For this review, take the finished solid that the model builds, in its own axes (mm). Face numbers are marked on the shaded views. A direction names the side the tool comes from. Give positions to 0.01 mm unless a question says otherwise; leave off trailing zeros. Order: outer loops, then holes, each group sorted by start corner. A loop starts at its lowest first (then second) coordinate and runs counter-clockwise, first axis right, second up. Notation, with made-up numbers: (46.25, 45.5) - (56.25, 45.5) arc R24 cw to (56.25, 65.5) - close; hole circle Ø11 at (84, 30.5). An arc over 180 degrees is marked (long way). One line per item, written item: value.
```python
from build123d import *

# Parameters (mm, degrees)
SKETCH_1_R                   = 36
EXTRUDE_1_DEPTH              = 26.5
CUT_EXTRUDE_3_DEPTH          = 58.395557319
CUT_EXTRUDE_3_DEPTH_BACK     = 58.395557319
SKETCH_5_R                   = 24
CUT_EXTRUDE_4_DEPTH          = 74.491496107
CUT_EXTRUDE_4_DEPTH_BACK     = 74.491496107
CUT_EXTRUDE_2_DEPTH          = 21.5
HOLE_WIZARD_M3_1_D           = 3.4
HOLE_WIZARD_M3_1_DEPTH       = 5
HOLE_WIZARD_M3_1_CBORE_D     = 6.5
HOLE_WIZARD_M3_1_CBORE_DEPTH = 3
PATTERN_CIRCULAR_1_COUNT     = 2
PATTERN_CIRCULAR_1_ANGLE     = 45
F_1_THE_OTHER_WAY_COUNT      = 2
F_1_THE_OTHER_WAY_ANGLE      = 45
MIRROR_1_COPY_1_D            = 3.4
MIRROR_1_COPY_1_DEPTH        = 5
MIRROR_1_COPY_1_CBORE_D      = 6.5
MIRROR_1_COPY_1_CBORE_DEPTH  = 3
MIRROR_1_COPY_2_D            = 3.4
MIRROR_1_COPY_2_DEPTH        = 5
MIRROR_1_COPY_2_CBORE_D      = 6.5
MIRROR_1_COPY_2_CBORE_DEPTH  = 3
FILLET_1_R                   = 5
SKETCH_10_R                  = 17.5
EXTRUDE_2_DEPTH              = 5
SKETCH_17_R                  = 15
EXTRUDE_3_DEPTH              = 7


with BuildPart() as part:
    # ｽｹｯﾁ1 → ﾎﾞｽ - 押し出し1 (new, symmetric)
    with BuildSketch(Plane.XY):
        Circle(SKETCH_1_R)
    extrude(amount=EXTRUDE_1_DEPTH, both=True)

    # ｽｹｯﾁ5 → ｶｯﾄ - 押し出し3 (cut, two sides: drawn at the far end of the back side and taken through both)
    with BuildSketch(Plane.XY.offset(-CUT_EXTRUDE_3_DEPTH_BACK)):
        Circle(SKETCH_5_R)
    extrude(amount=CUT_EXTRUDE_3_DEPTH + CUT_EXTRUDE_3_DEPTH_BACK, mode=Mode.SUBTRACT)

    # ｽｹｯﾁ6 → ｶｯﾄ - 押し出し4 (cut, two sides: drawn at the far end of the back side and taken through both)
    with BuildSketch(Plane.XY.offset(26.5).offset(-CUT_EXTRUDE_4_DEPTH_BACK)):
        with BuildLine():
            Line((-33.25966317, 13.776603565), (0, 0))
            Line((0, 0), (33.25966317, 13.776603565))
            ThreePointArc((33.25966317, 13.776603565), (0, -36), (-33.25966317, 13.776603565))
        make_face()
    extrude(amount=CUT_EXTRUDE_4_DEPTH + CUT_EXTRUDE_4_DEPTH_BACK, mode=Mode.SUBTRACT)

    # ｽｹｯﾁ3 → ｶｯﾄ - 押し出し2 (cut, symmetric)
    with BuildSketch(Plane.XY):
        with BuildLine():
            Line((-33.25966317, 13.776603565), (-28.640265508, 11.863186403))
            ThreePointArc((-28.640265508, 11.863186403), (0, 31), (28.640265508, 11.863186403))
            Line((28.640265508, 11.863186403), (33.25966317, 13.776603565))
            ThreePointArc((33.25966317, 13.776603565), (0, -36), (-33.25966317, 13.776603565))
        make_face()
    extrude(amount=CUT_EXTRUDE_2_DEPTH, both=True, mode=Mode.SUBTRACT)

    # M3 穴付きねじ用座ぐり穴1
    with Locations(Plane.XY.offset(26.5)):
        with Locations((0, 27.5)):
            hole_wizard_m3_1 = CounterBoreHole(HOLE_WIZARD_M3_1_D / 2, HOLE_WIZARD_M3_1_CBORE_D / 2, HOLE_WIZARD_M3_1_CBORE_DEPTH, depth=HOLE_WIZARD_M3_1_DEPTH)

    # 円形ﾊﾟﾀｰﾝ1: M3 穴付きねじ用座ぐり穴1 ×2 about axis
    pattern_circular_1_axis = Axis((0, 0, 26.5), (0, 0, -1))
    for i in range(1, PATTERN_CIRCULAR_1_COUNT):
        add(hole_wizard_m3_1.rotate(pattern_circular_1_axis, i * PATTERN_CIRCULAR_1_ANGLE / (PATTERN_CIRCULAR_1_COUNT - 1)), mode=Mode.SUBTRACT)

    # 1 the other way: M3 穴付きねじ用座ぐり穴1 ×2 about axis
    f_1_the_other_way_axis = Axis((0, 0, 26.5), (0, 0, 1))
    for i in range(1, F_1_THE_OTHER_WAY_COUNT):
        add(hole_wizard_m3_1.rotate(f_1_the_other_way_axis, i * F_1_THE_OTHER_WAY_ANGLE / (F_1_THE_OTHER_WAY_COUNT - 1)), mode=Mode.SUBTRACT)

    # ﾐﾗｰ1: M3 穴付きねじ用座ぐり穴1 across plane
    add(hole_wizard_m3_1.mirror(Plane.XY), mode=Mode.SUBTRACT)

    # ﾐﾗｰ1 copy 1
    with Locations(Plane(origin=(0, 0, -26.5), x_dir=(0.7071067811865462, -0.7071067811865488, 0), z_dir=(0, 0, -1))):
        with Locations((0, -27.5)):
            CounterBoreHole(MIRROR_1_COPY_1_D / 2, MIRROR_1_COPY_1_CBORE_D / 2, MIRROR_1_COPY_1_CBORE_DEPTH, depth=MIRROR_1_COPY_1_DEPTH)

    # ﾐﾗｰ1 copy 2
    with Locations(Plane(origin=(0, 0, -26.5), x_dir=(0.7071067811865462, 0.7071067811865488, 0), z_dir=(0, 0, -1))):
        with Locations((0, -27.5)):
            CounterBoreHole(MIRROR_1_COPY_2_D / 2, MIRROR_1_COPY_2_CBORE_D / 2, MIRROR_1_COPY_2_CBORE_DEPTH, depth=MIRROR_1_COPY_2_DEPTH)

    # ﾌｨﾚｯﾄ1
    # the kernel refuses this fillet: 5 mm, written as the material it takes off along each edge
    with BuildSketch(Plane(origin=(33.25966317, 13.776603565, 41.063878514), x_dir=(-0.4561802532309845, 0.88988739543951, 0), z_dir=(0, 0, -1)), Plane(origin=(-33.25966317, 13.776603565, -41.063878514), x_dir=(0.45618025323098454, 0.88988739543951, 0), z_dir=(0, 0, 1))) as fillet_1_piece_1:
        with BuildLine():
            CenterArc((5.420999225, -4.98360688), FILLET_1_R, 85.359100457, 99.281799087)
            Line((0.437392345, -5.388159061), (0, 0))
            ThreePointArc((0, 0), (2.912775703, 0.118030465), (5.825551406, 0))
        make_face()
    extrude(amount=82.127757029, mode=Mode.SUBTRACT)
    with BuildSketch(Plane(origin=(22.17310878, 9.184402377, -37.914284285), x_dir=(0.9238795325112864, 0.38268343236509056, 0), z_dir=(0, 0, 1)), Plane(origin=(22.17310878, 9.184402377, 10.085715715), x_dir=(0.9238795325112864, 0.38268343236509056, 0), z_dir=(0, 0, 1))) as fillet_1_piece_2:
        with BuildLine():
            CenterArc((4.565713714, 5), FILLET_1_R, 189.928191842, 80.071808158)
            ThreePointArc((-0.35940934, 4.137931034), (-0.090021164, 2.076755181), (0, 0))
            Line((0, 0), (4.565713714, 0))
        make_face()
    extrude(amount=27.828568571, mode=Mode.SUBTRACT)
    with BuildSketch(Plane(origin=(-22.17310878, 9.184402377, -37.914284285), x_dir=(-0.9238795325112864, 0.38268343236509056, 0), z_dir=(0, 0, 1)), Plane(origin=(-22.17310878, 9.184402377, 10.085715715), x_dir=(-0.9238795325112864, 0.38268343236509056, 0), z_dir=(0, 0, 1))) as fillet_1_piece_3:
        with BuildLine():
            CenterArc((4.565713714, -5), FILLET_1_R, 90, 80.071808158)
            ThreePointArc((-0.35940934, -4.137931034), (-0.090021164, -2.076755181), (0, 0))
            Line((0, 0), (4.565713714, 0))
        make_face()
    extrude(amount=27.828568571, mode=Mode.SUBTRACT)

    # ｽｹｯﾁ10 → ﾎﾞｽ - 押し出し2 (add, through all)
    with BuildSketch(Plane(origin=(0, 31, 0), x_dir=(-1, 0, 0), z_dir=(0, -1, 0))):
        Circle(SKETCH_10_R)
    extrude(amount=-EXTRUDE_2_DEPTH)

    # ｽｹｯﾁ17 → ﾎﾞｽ - 押し出し3 (add)
    with BuildSketch(Plane(origin=(0, 36, 0), x_dir=(1, 0, 0), z_dir=(0, 1, 0))):
        with Locations(Location((0, 0, 0), (0, 0, 90))):
            Circle(SKETCH_17_R)
    extrude(amount=EXTRUDE_3_DEPTH)


solid = part.part
```
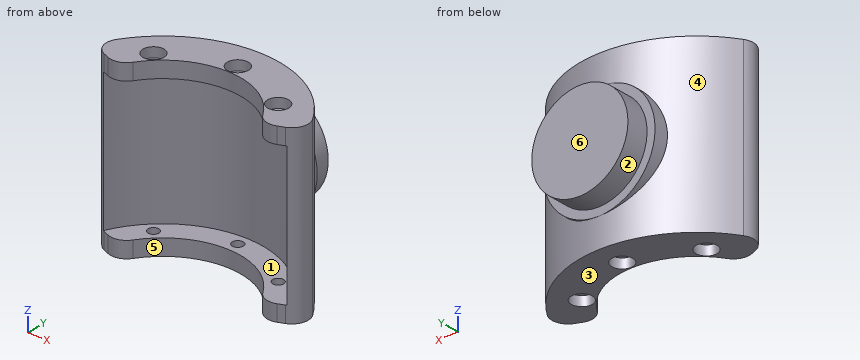
(1) Take a section at A-A (z = 0). Write out the cut boundary in (x, y), then the cut area to 3 significant figures.
Answers below:
outline: (-30.6, 18.96) arc R5 ccw to (-28.63, 11.88) arc R31 cw to (28.63, 11.88) arc R5 ccw to (30.6, 18.96) arc R36 ccw to (17.5, 31.46) - (17.5, 36) - (15, 36) - (15, 43) - (-15, 43) - (-15, 36) - (-17.5, 36) - (-17.5, 31.46) arc R36 ccw to start
area: 643 mm^2
(2) Take a section at D-D (y = 39). Write out the cut boundary in (x, z).
Answers below:
outline: circle Ø30 at (0, 0)
(3) Wall thickness on line 1 (Z direction, x = -7, y = 27.5); line 2 (Y direction, x = 0, z = 22.6); line 3 (Y direction, x = 0, z = 24.55): over which ranges is each line inside the solid? List them lowest first. Write a range as from..to.
Answers below:
line 1: z = -26.5..-21.5, 21.5..26.5
line 2: y = 24..25.8, 29.2..36
line 3: y = 24..24.25, 30.75..36
(4) Machinability: for the marked faces 1, 2 and 3, which of the approach directions +Z, -Z, +X, -X, +Y, -Y give a long, thin tool a straight path to every point of the face, cutting with its end or side? Answer none if there is none.
Answers below:
face 1: -Y
face 2: +Y
face 3: -Z, +X, -X, +Y, -Y
(5) Take a section at C-C (x = -8.5). Write out the cut boundary in (y, z), then the cut area to 3 significant figures.
Answers below:
outline: (22.44, -26.5) - (34.98, -26.5) - (34.98, -15.3) - (36, -15.3) - (36, -12.36) - (43, -12.36) - (43, 12.36) - (36, 12.36) - (36, 15.3) - (34.98, 15.3) - (34.98, 26.5) - (22.44, 26.5) - (22.44, 21.5) - (29.81, 21.5) - (29.81, -21.5) - (22.44, -21.5) - close
area: 552 mm^2
(6) For P1, Ø2.5, axis at x = 0, y = 27.5, coming from the -Z side; P2, Ø1.5, axis at x = 7, y = 38, coming from the +Z side; P3, Ø6, axis at x = -19.45, y = 19.45, coming from the +Z side; P4, Ø4, axis at x = 19.45, y = 19.45, coming from the -Z side, all flat-tipped, find the tip position at first contact; note any pin that passes through.
Answers below:
P1: passes through
P2: stops at z = 13.64
P3: stops at z = 23.5
P4: stops at z = -23.5
(7) Take a section at B-B (y = 27.5). Write out the cut boundary in (x, z), then the cut area to 3 significant figures.
Answers below:
outline: (-23.23, -26.5) - (-3.25, -26.5) - (-3.25, -23.5) - (-1.7, -23.5) - (-1.7, -21.5) - (-14.31, -21.5) - (-14.31, 21.5) - (-1.7, 21.5) - (-1.7, 23.5) - (-3.25, 23.5) - (-3.25, 26.5) - (-23.23, 26.5) - close; (1.7, -23.5) - (3.25, -23.5) - (3.25, -26.5) - (23.23, -26.5) - (23.23, 26.5) - (3.25, 26.5) - (3.25, 23.5) - (1.7, 23.5) - (1.7, 21.5) - (14.31, 21.5) - (14.31, -21.5) - (1.7, -21.5) - close
area: 1,180 mm^2
(8) Draft analysis for pull direction X (two halves, no side actions). For the marked faces 4, 5 and 6, state which applies: pulls with the +X half, pulls with the -X half, needs draft (parallel to the pull), parting line crosses it, or undercut.
Answers below:
face 4: parting line crosses it
face 5: undercut
face 6: needs draft
